Part model, mm, in its own coordinate system. A direction names the side the tool comes from. Coordinates: 2 decimals unless noted, no trailing zeros. Order: outer loops, then holes, each group sorted by start corner. A loop starts at its lowest first (then second) coordinate and runs counter-clockwise, first axis right, second up. Notation, with made-up numbers: (43.25, -21.5) - (53.25, -21.5) arc R12 ccw to (53.25, -3.5) - close; hole circle Ø10 at (48.5, 36.25). An arc over 180 degrees is marked (long way). Use a Markdown table: item, result. Add a question column.
1) Tool access for faces 1 (the face through (-18.5, 6.3, 2.5)), 2 (the face through (-16.3, 0, 9.3)), 3 (the face through (2.343, 17.847, 0.986)): list every direction of +Z, -Z, +X, -X, +Y, -Y with a clear straight run to the whole face (end or side of a thin tool).
2) Saw through at C-C on y = -8.75. List the corners of the cut face in (x, z).
3) Saw through at B-B on x = 15. List the corners of the cut face in (y, z), then the cut area to 3 significant figures.
4) Drop flat-ended pins along their axis: P1, Ø5, axis at x = -2, z = 10, coming from the +Y side; P2, Ø2, axis at y = -6.5, z = 7, coming from the -X side; P3, Ø2.5, axis at x = -7.5, y = 12.99, coming from the -Z side; P4, Ø5, axis at y = 15, z = 9, coming from the +X side. Give the stop position or say it passes through.
5) Two-plate mould, pull along Y, no slides. Class faces 4 (the face through (17.31, 4.93, 8.45)), 5 (the face through (17, -8, 5)), 6 (the face through (-18.5, -8.7, 2.5)): +Y half, -Y half, draft (parallel to the pull), parting line (faces both ways), or undercut.
6) Wall check: L1, parallel to Y at x = 0, z = 1.5; L2, parallel to Z at x = 9.5, y = 13.5; L3, parallel to Z at x = -15, y = -21. Give the ranges that are in metal, low to high. Write a range as [from, to].
7) Saw through at A-A on z = 8. List the corners of the cut face in (x, y).
8) Saw through at D-D on x = 31.5. List the corners of the cut face in (y, z), then the cut area to 3 significant figures.
```python
from build123d import *

# Parameters (mm, degrees)
SKETCH1_R           = 40
BOSS_EXTRUDE1_DEPTH = 5
SKETCH2_R           = 18
BOSS_EXTRUDE2_DEPTH = 7
CUT_EXTRUDE1_REACH  = 59.827
SKETCH3_R           = 13
SKETCH5_W           = 3.5
SKETCH5_H           = 10.665364504
CUT_EXTRUDE3_DEPTH  = 7
SKETCH6_R           = 1.25
CUT_EXTRUDE4_DEPTH  = 58
SKETCH8_R           = 1.5
CUT_EXTRUDE5_DEPTH  = 58.827329179
CIRPATTERN1_COUNT   = 3
SKETCH10_R          = 1.5
CUT_EXTRUDE6_DEPTH  = 58.827329179
SKETCH11_OUTSIDE_W  = 104.754
SKETCH11_OUTSIDE_H  = 104.754
SKETCH11_OUTSIDE_R  = 25
CUT_EXTRUDE8_DEPTH  = 3
SKETCH12_R          = 18
CUT_EXTRUDE9_DEPTH  = 2
SKETCH13_R          = 1
CUT_EXTRUDE10_DEPTH = 58.827329179


with BuildPart() as part:
    # Sketch1 → Boss-Extrude1 (new body)
    with BuildSketch(Plane.XY):
        Circle(SKETCH1_R)
    extrude(amount=BOSS_EXTRUDE1_DEPTH)

    # Sketch2 → Boss-Extrude2 (add)
    with BuildSketch(Plane.XY.offset(5)):
        Circle(SKETCH2_R)
    extrude(amount=BOSS_EXTRUDE2_DEPTH)

    # Sketch3 → Cut-Extrude1 (cut, up to next)
    with BuildSketch(Plane.XY.offset(12), mode=Mode.PRIVATE) as cut_extrude1_sk1:
        Circle(SKETCH3_R)
    cut_extrude1_tool1 = extrude(cut_extrude1_sk1.sketch, amount=-CUT_EXTRUDE1_REACH, mode=Mode.PRIVATE) & part.part
    add(cut_extrude1_tool1.solids().sort_by_distance((0, 0, 12))[0], mode=Mode.SUBTRACT)

    # Sketch5 → Cut-Extrude3 (cut)
    with BuildSketch(Plane.XY.offset(12)):
        with Locations((-16.25, -5.332682252)):
            Rectangle(SKETCH5_W, SKETCH5_H)
    extrude(amount=-CUT_EXTRUDE3_DEPTH, mode=Mode.SUBTRACT)

    # Sketch6 → Cut-Extrude4 (cut, through all)
    with BuildSketch(Plane.XY.offset(5)):
        with Locations((-16, -1.25)):
            Circle(SKETCH6_R)
    extrude(amount=-CUT_EXTRUDE4_DEPTH, mode=Mode.SUBTRACT)

    # Sketch8 → Cut-Extrude5 (cut, through all)
    with BuildSketch(Plane.XY.offset(12)):
        with Locations((15, 0)):
            Circle(SKETCH8_R)
    cut_extrude5 = extrude(amount=-CUT_EXTRUDE5_DEPTH, mode=Mode.SUBTRACT)

    # CirPattern1: Cut-Extrude5 ×3 about axis
    cirpattern1_axis = Axis((0, 0, 0), (0, 0, 1))
    for i in range(1, CIRPATTERN1_COUNT):
        add(cut_extrude5.rotate(cirpattern1_axis, i * 360 / CIRPATTERN1_COUNT), mode=Mode.SUBTRACT)

    # Sketch10 → Cut-Extrude6 (cut, through all)
    with BuildSketch(Plane(origin=(0, 0, 0), x_dir=(-1, 0, 0), z_dir=(0, 0, -1))):
        with Locations((20, 6.25)):
            Circle(SKETCH10_R)
        with Locations((20, -8.75)):
            Circle(SKETCH10_R)
    extrude(amount=-CUT_EXTRUDE6_DEPTH, mode=Mode.SUBTRACT)

    # Sketch11 outside → Cut-Extrude8 (cut)
    with BuildSketch(Plane(origin=(0, 0, 0), x_dir=(-1, 0, 0), z_dir=(0, 0, -1))):
        Rectangle(SKETCH11_OUTSIDE_W, SKETCH11_OUTSIDE_H)
        Circle(SKETCH11_OUTSIDE_R, mode=Mode.SUBTRACT)
    extrude(amount=-CUT_EXTRUDE8_DEPTH, mode=Mode.SUBTRACT)

    # Sketch12 → Cut-Extrude9 (cut)
    with BuildSketch(Plane(origin=(0, 0, 0), x_dir=(-1, 0, 0), z_dir=(0, 0, -1))):
        Circle(SKETCH12_R)
    extrude(amount=-CUT_EXTRUDE9_DEPTH, mode=Mode.SUBTRACT)

    # Sketch13 → Cut-Extrude10 (cut, through all)
    with BuildSketch(Plane.XZ):
        with Locations(Location((-16, 8, 0), (0, 0, 270))):
            Circle(SKETCH13_R)
    extrude(amount=-CUT_EXTRUDE10_DEPTH, mode=Mode.SUBTRACT)


solid = part.part
```
Results are:
| question | item | result |
|---|---|---|
| 1 | face 1 | +Z, -Z |
| 1 | face 2 | +Z, -X, -Y |
| 1 | face 3 | -Z |
| 2 | outline | (-39.03, 3) - (-23.42, 3) - (-23.42, 0) - (-21.5, 0) - (-21.5, 5) - (-39.03, 5) - close; (-18.5, 0) - (-15.73, 0) - (-15.73, 2) - (-9.61, 2) - (-9.61, 12) - (-14.5, 12) - (-14.5, 5) - (-18.5, 5) - close; (9.61, 2) - (15.73, 2) - (15.73, 0) - (23.42, 0) - (23.42, 3) - (39.03, 3) - (39.03, 5) - (15.73, 5) - (15.73, 12) - (9.61, 12) - close |
| 3 | outline | (-37.08, 3) - (-20, 3) - (-20, 0) - (-9.95, 0) - (-9.95, 2) - (-1.5, 2) - (-1.5, 12) - (-9.95, 12) - (-9.95, 5) - (-37.08, 5) - close; (1.5, 2) - (9.95, 2) - (9.95, 0) - (20, 0) - (20, 3) - (37.08, 3) - (37.08, 5) - (9.95, 5) - (9.95, 12) - (1.5, 12) - close |
| 3 | area | 338 mm2 |
| 4 | P1 | y = 18 |
| 4 | P2 | x = -14.5 |
| 4 | P3 | through |
| 4 | P4 | x = 12.95 |
| 5 | face 4 | parting line |
| 5 | face 5 | draft |
| 5 | face 6 | undercut |
| 6 | L1 | [-25, -18], [18, 25] |
| 6 | L2 | [2, 12] |
| 6 | L3 | [3, 5] |
| 7 | outline | (-18, 0) - (-17, 0) - (-17, 5.92) arc R18 ccw to start; (-15, 0) - (-14.5, 0) - (-14.5, -10.67) arc R18 ccw (long way) to (-15, 9.95) - close; hole circle Ø26 at (0, 0); hole circle Ø3 at (-7.5, -12.99); hole circle Ø3 at (-7.5, 12.99); hole circle Ø3 at (15, 0) |
| 8 | outline | (-24.65, 3) - (24.65, 3) - (24.65, 5) - (-24.65, 5) - close |
| 8 | area | 98.6 mm2 |
